from build123d import *

# Parameters (mm, degrees)
BASPROSKE_W                = 8.6
BASPROSKE_H                = 3
TOOTHCUT_DEPTH             = 10.589577676
TEETHCUTS_COUNT            = 10
BORSKE_R                   = 0.4
BORE_DEPTH                 = 50.0000508
SKETCH1_R                  = 8
BOSS_EXTRUDE1_DEPTH        = 2.5
M1_6_CLEARANCE_HOLE1_D     = 1.8
M1_6_CLEARANCE_HOLE1_DEPTH = 4.25
M1_6_CLEARANCE_HOLE1_TIP   = 0.540774557


with BuildPart() as part:
    # BasProSke → Base-Revolve (revolve)
    with BuildSketch(Plane(origin=(0, 0, 0), x_dir=(1, 0, 0), z_dir=(0, 1, 0)), mode=Mode.PRIVATE) as base_revolve_sk:
        with Locations((4.3, 1.5)):
            Rectangle(BASPROSKE_W, BASPROSKE_H)
    revolve(base_revolve_sk.sketch.rotate(Axis((-10, 0, 0), (1, 0, 0)), 180), axis=Axis((-10, 0, 0), (1, 0, 0)))

    # TooCutSke → ToothCut (cut, through all)
    with BuildSketch(Plane(origin=(0, 0, 0), x_dir=(0, 0, -1), z_dir=(1, 0, 0))):
        with BuildLine():
            ThreePointArc((0.296449938, 1.850403587), (0, 1.874), (-0.296449938, 1.850403587))
            ThreePointArc((-0.296449938, 1.850403587), (-0.428089565, 2.470295585), (-0.905889751, 2.886591228))
            ThreePointArc((-0.905889751, 2.886591228), (0, 3.0254), (0.905889751, 2.886591228))
            ThreePointArc((0.905889751, 2.886591228), (0.428089565, 2.470295585), (0.296449938, 1.850403587))
        make_face()
    toothcut = extrude(amount=TOOTHCUT_DEPTH, mode=Mode.SUBTRACT)

    # TeethCuts: ToothCut ×10 about axis
    teethcuts_axis = Axis((0, 0, 0), (1, 0, 0))
    for i in range(1, TEETHCUTS_COUNT):
        add(toothcut.rotate(teethcuts_axis, i * 360 / TEETHCUTS_COUNT), mode=Mode.SUBTRACT)

    # BorSke → Bore (cut, symmetric)
    with BuildSketch(Plane(origin=(0, 0, 0), x_dir=(0, 0, -1), z_dir=(1, 0, 0))):
        with Locations(Location((0, 0, 0), (0, 0, 180))):
            Circle(BORSKE_R)
    extrude(amount=BORE_DEPTH, both=True, mode=Mode.SUBTRACT)

    # Sketch1 → Boss-Extrude1 (add)
    with BuildSketch(Plane.ZY):
        Circle(SKETCH1_R)
    extrude(amount=-BOSS_EXTRUDE1_DEPTH)

    # M1.6 Clearance Hole1
    with Locations(Plane(origin=(2.5, 0, 0), x_dir=(0, 0, -1), z_dir=(1, 0, 0))):
        with Locations((0, 6), (6, 0), (0, -6), (-6, 0)):
            Hole(M1_6_CLEARANCE_HOLE1_D / 2, depth=M1_6_CLEARANCE_HOLE1_DEPTH)
            with Locations((0, 0, -(M1_6_CLEARANCE_HOLE1_DEPTH + M1_6_CLEARANCE_HOLE1_TIP / 2))):  # 118° drill point
                Cone(0, M1_6_CLEARANCE_HOLE1_D / 2, M1_6_CLEARANCE_HOLE1_TIP, mode=Mode.SUBTRACT)


solid = part.part
Input: part model. Units: mm. Frame: model coordinates. Round coordinates to 2 decimals unless told otherwise and drop trailing zeros. Order: outer loops, then holes, each group sorted by start corner. A loop starts at its lowest first (then second) coordinate and runs counter-clockwise, first axis right, second up. Notation, with made-up numbers: (44, 7) - (60, 7) arc R16 ccw to (60, 24) - close; hole circle Ø5 at (23, -18.75). An arc over 180 degrees is marked (long way). Use a Markdown table: item, result.
1. Section A-A on z = 0. Return the cut outline in (x, y).
Evaluation:
| item | result |
|---|---|
| outline | (0, -8) - (2.5, -8) - (2.5, -6.9) - (0, -6.9) - close; (0, -5.1) - (2.5, -5.1) - (2.5, -1.87) - (8.6, -1.87) - (8.6, -0.4) - (2.5, -0.4) - (2.5, 0.4) - (8.6, 0.4) - (8.6, 1.87) - (2.5, 1.87) - (2.5, 5.1) - (0, 5.1) - close; (0, 6.9) - (2.5, 6.9) - (2.5, 8) - (0, 8) - close |
2. First-contact query: pin 1 (0.6 mm diameter, centred on y = 0, z = 0, fed in from +X); pin 2 (4 mm diameter, centred on x = 6, z = 4.5, fed in from -Y); pin 3 (4 mm diameter, centred on x = 1.5, y = 3, fed in from -Z). Flat tips, straight axial feed; report the tip coordinate or a pass-through.
Evaluation:
| item | result |
|---|---|
| pin 1 | x = 2.5 |
| pin 2 | y = -0.35 |
| pin 3 | z = -7.94 |
3. Section C-C on y = -6.5. Return the cut outline in (x, z).
Evaluation:
| item | result |
|---|---|
| outline | (0, -4.66) - (2.5, -4.66) - (2.5, -0.75) - (0, -0.75) - close; (0, 0.75) - (2.5, 0.75) - (2.5, 4.66) - (0, 4.66) - close |
4. Section D-D on z = -6.25. Return the cut outline in (x, y), then the cut area to 3 significant figures.
Evaluation:
| item | result |
|---|---|
| outline | (0, -4.99) - (2.5, -4.99) - (2.5, -0.86) - (0, -0.86) - close; (0, 0.86) - (2.5, 0.86) - (2.5, 4.99) - (0, 4.99) - close |
| area | 20.6 mm^2 |
5. Material intervals for probe 1 along Y at (x, z) = (1.7, 0); probe 2 along Y at (x, z) = (4.75, 0); probe 3 along Z at (x, y) = (6.5, 0.75), sorted ascending.
Evaluation:
| item | result |
|---|---|
| probe 1 | -8 to -6.9, -5.1 to 5.1, 6.9 to 8 |
| probe 2 | -1.87 to -0.4, 0.4 to 1.87 |
| probe 3 | -1.72 to 1.72 |
6. Section B-B on x = 2. Return the cut outline in (y, z).
Evaluation:
| item | result |
|---|---|
| outline | circle Ø16 at (0, 0); hole circle Ø1.8 at (-6, 0); hole circle Ø1.8 at (0, -6); hole circle Ø1.8 at (0, 6); hole circle Ø1.8 at (6, 0) |
